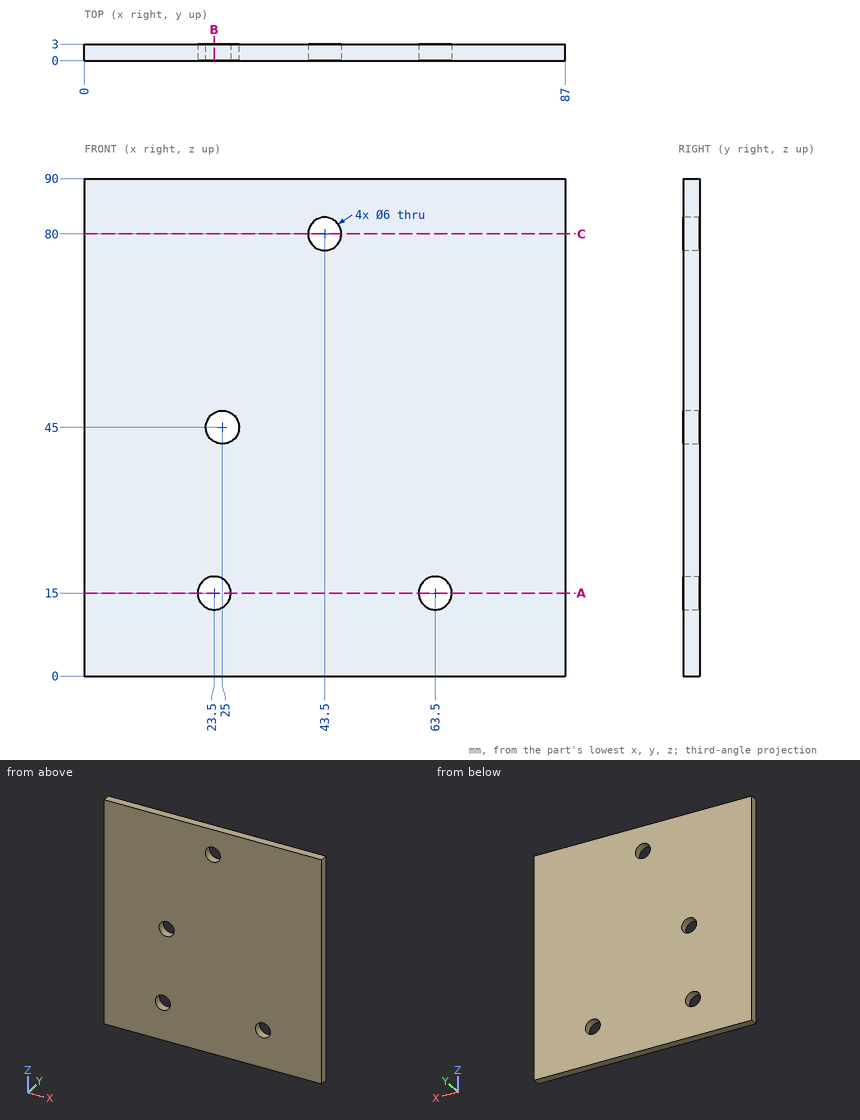
Can you work these out from the drawing? Everything is in mm from the part's minimum corner. Coordinates: 2 decimals unless noted, no trailing zeros. Loops run counter-clockwise (first coordinate to the right, second up) from the corner with the lowest first, then second, coordinate; pieces in that order, holes last. Notation, with made-up numbers: (-38.75, 11.5) - (-16.75, 11.5) arc R16 ccw to (-16.75, 38.5) - close; hole circle Ø3 at (7.25, 62.25). An arc over 180 degrees is marked (long way). Put each result on its own line as item: value. Start each with the question number.
Item 1: Suppose I cut it at C-C (z = 80). Please give me the cut outline in (x, y), and give its area (3 significant figures).
Item 2: For pin 1 (5 mm diameter, centred on x = 43.5, z = 80, fed in from -Y), with a flat end and sliding along its axis, tell me the tip position at first contact or that it passes through.
Item 3: Suppose I cut it at B-B (x = 23.5). Please give me the cut outline in (y, z).
Item 4: Suppose I cut it at A-A (z = 15). Please give me the cut outline in (x, y), and give its area (3 significant figures).
Item 5: If I drill on line 1 along X through (y, z) = (1.7, 15); line 2 along X through (y, z) = (1.9, 80); line 3 along X through (y, z) = (1, 45), over which ranges is the centre line in solid material (lowest first)?
Here are the results:
1. outline: (0, 0) - (40.5, 0) - (40.5, 3) - (0, 3) - close; (46.5, 0) - (87, 0) - (87, 3) - (46.5, 3) - close
1. area: 243 mm²
2. pin 1: through
3. outline: (0, 0) - (3, 0) - (3, 12) - (0, 12) - close; (0, 18) - (3, 18) - (3, 42.4) - (0, 42.4) - close; (0, 47.6) - (3, 47.6) - (3, 90) - (0, 90) - close
4. outline: (0, 0) - (20.5, 0) - (20.5, 3) - (0, 3) - close; (26.5, 0) - (60.5, 0) - (60.5, 3) - (26.5, 3) - close; (66.5, 0) - (87, 0) - (87, 3) - (66.5, 3) - close
4. area: 225 mm²
5. line 1: 0 to 20.5, 26.5 to 60.5, 66.5 to 87
5. line 2: 0 to 40.5, 46.5 to 87
5. line 3: 0 to 22, 28 to 87
